Verification items for the finished model (mm, model axes). Face numbers are marked on the shaded views. Give positions to 0.01 mm unless a question says otherwise; leave off trailing zeros. Write each loop counter-clockwise with the first axis right and the second up, starting at its lowest first coordinate (ties: lowest second). Pieces come first, ordered by that corner, then holes. Notation, with made-up numbers: M -38.75,-26.5 L 10.25,-26.5 A33 cw 10.25,1.5 Z; hole C -30.75,-30.5 d9. An arc over 180 degrees is marked long. Write item = value, one per line.
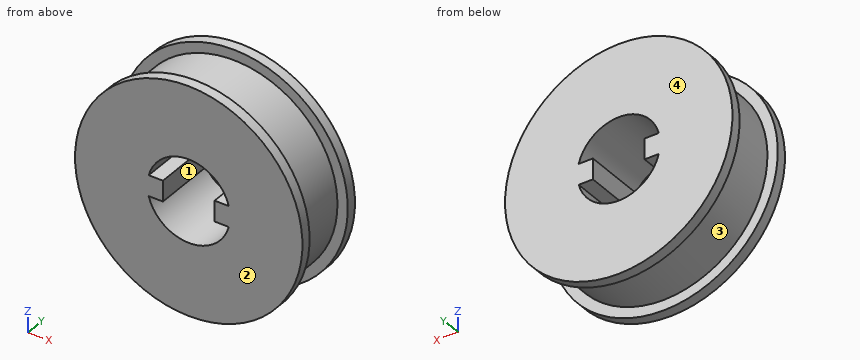
from build123d import *

# Parameters (mm, degrees)
ESQUISSE6_W        = 4.5
ESQUISSE6_H        = 3
BOSS_EXTRU_1_DEPTH = 11


with BuildPart() as part:
    # Esquisse2 → Révolution1 (revolve)
    with BuildSketch(Plane.XY, mode=Mode.PRIVATE) as r_volution1_sk:
        Polygon((6, 5.365286165), (6, -5.634713835), (16.5, -5.634713835), (16.5, -4.134713835), (15, -4.134713835), (15, 3.865286165), (16.5, 3.865286165), (16.5, 5.365286165), align=None)
    revolve(r_volution1_sk.sketch.rotate(Axis((0, 0, 0), (0, 1, 0)), 90), axis=Axis((0, 0, 0), (0, 1, 0)))

    # Esquisse6 → Boss.-Extru.1 (add)
    with BuildSketch(Plane(origin=(0, 5.365286165, 0), x_dir=(1, 0, 0), z_dir=(0, 1, 0))):
        with Locations((-6, 0)):
            Rectangle(ESQUISSE6_W, ESQUISSE6_H)
        with Locations((6, 0)):
            Rectangle(ESQUISSE6_W, ESQUISSE6_H)
    extrude(amount=-BOSS_EXTRU_1_DEPTH)


solid = part.part
1) Cross-section at C-C on x = 0. Record the boundary of the cut face in (y, z).
From the geometry:
outline = M -5.63,-16.5 L -4.13,-16.5 L -4.13,-15 L 3.87,-15 L 3.87,-16.5 L 5.37,-16.5 L 5.37,-6 L -5.63,-6 Z; M -5.63,6 L 5.37,6 L 5.37,16.5 L 3.87,16.5 L 3.87,15 L -4.13,15 L -4.13,16.5 L -5.63,16.5 Z
2) Depth check by flat-ended pin: P1, Ø1, axis at x = 12.5, y = 1, coming from the +Z side; P2, Ø1, axis at x = 4.5, y = 0, coming from the -Z side; P3, Ø0.9, axis at y = 0.5, z = 0, coming from the -X side. Enter the tip coordinate at first touch or a pass-through.
From the geometry:
P1 = 9
P2 = -14.46
P3 = -15
3) Cross-section at D-D on z = -10.5. Record the boundary of the cut face in (x, y).
From the geometry:
outline = M -12.73,-5.63 L 12.73,-5.63 L 12.73,-4.13 L 10.71,-4.13 L 10.71,3.87 L 12.73,3.87 L 12.73,5.37 L -12.73,5.37 L -12.73,3.87 L -10.71,3.87 L -10.71,-4.13 L -12.73,-4.13 Z
4) Draft check along Y on the marked faces 1, 2, 3 and 4. Enter one of: +Y half, -Y half, draft (parallel to the pull), parting line (faces both ways), or undercut.
From the geometry:
face_1 = draft
face_2 = -Y half
face_3 = undercut
face_4 = +Y half
5) Cross-section at A-A on z = 0. Record the boundary of the cut face in (x, y).
From the geometry:
outline = M -16.5,-5.63 L -3.75,-5.63 L -3.75,5.37 L -16.5,5.37 L -16.5,3.87 L -15,3.87 L -15,-4.13 L -16.5,-4.13 Z; M 3.75,-5.63 L 16.5,-5.63 L 16.5,-4.13 L 15,-4.13 L 15,3.87 L 16.5,3.87 L 16.5,5.37 L 3.75,5.37 Z
6) Material ranges on probe 1 along Y at (x, z) = (-11.5, 11); probe 2 along X at (y, z) = (-4.25, -0.5); probe 3 along X at (y, z) = (-1.75, 4), recorded low to high. Write a range as from..to.
From the geometry:
probe_1 = -5.63..-4.13, 3.87..5.37
probe_2 = -16.49..-3.75, 3.75..16.49
probe_3 = -14.46..-4.47, 4.47..14.46
7) Cross-section at B-B on y = -3. Record the boundary of the cut face in (x, z).
From the geometry:
outline = C 0,0 d30; hole M -5.81,-1.5 A6 ccw 5.81,-1.5 L 3.75,-1.5 L 3.75,1.5 L 5.81,1.5 A6 ccw -5.81,1.5 L -3.75,1.5 L -3.75,-1.5 Z
